from build123d import *

# Parameters (mm, degrees)
F0_W     = 85.001712665
F0_H     = 72.736363858
F1_DEPTH = 25.4
F2_R     = 5
F3_R     = 5


with BuildPart() as f1:
    # F0 (on Front) → F1 (new body)
    with BuildSketch(Plane.XZ):
        with Locations((-16.5439592674, 2.8524082154)):
            Rectangle(F0_W, F0_H)
    extrude(amount=F1_DEPTH)

    # F2
    f2_edges = [f1.edges().sort_by_distance(p)[0] for p in [
        (25.956897, -12.7, 39.22059),
    ]]
    fillet(f2_edges, radius=F2_R)

    # F3
    f3_edges = [f1.edges().sort_by_distance(p)[0] for p in [
        (25.956897, 0, 0.352408),
        (25.956897, -12.7, 34.22059),
        (25.956897, -12.7, -33.515774),
        (25.956897, -25.4, 0.352408),
        (20.956897, -12.7, 39.22059),
    ]]
    fillet(f3_edges, radius=F3_R)


solid = f1.part
Part model, mm, in its own coordinate system. Coordinates: 2 decimals unless noted, no trailing zeros. Loops run counter-clockwise (first coordinate to the right, second up) from the corner with the lowest first, then second, coordinate; pieces in that order, holes last. Notation, with made-up numbers: M 79,58 L 116,58 A33 ccw 116,90 Z; hole C 8,63.5 d7. An arc over 180 degrees is marked long. Use a Markdown table: item, result. Add a question column.
Q1. Cut at A-A (y = -23). Write the cut outline in (x, z).
Q2. Probe L1, parallel to X at y = -20.75, z = 18; L2, parallel to X at y = -22.5, z = -13; L3, parallel to Z at x = 22.5, y = -12.5. List the from-to ranges inside material, lowest first.
Q3. Pin check, flat tip, straight feed: P1, Ø5, axis at x = -49, y = -3.5, coming from the +Z side. Stop position of the tip, or through.
Worked out:
| question | item | result |
|---|---|---|
| 1 | outline | M -59.04,-33.52 L 20.96,-33.52 A5 ccw 25.23,-31.12 L 25.23,34.22 A4.27 ccw 20.96,38.49 L -59.04,38.49 Z |
| 2 | L1 | x = -59.04 to 25.94 |
| 2 | L2 | x = -59.04 to 25.49 |
| 2 | L3 | z = -33.27 to 38.98 |
| 3 | P1 | stops at z = 39.22 |
